from build123d import *

# Parameters (mm, degrees)
F0_W     = 463
F0_H     = 316
F1_DEPTH = 12
F3_DEPTH = 12.001
F4_W     = 408
F4_H     = 10
F4_W_2   = 391
F5_DEPTH = 5.75
F6_R     = 10
F7_R     = 5


with BuildPart() as f1:
    # F0 (on Top) → F1 (new body)
    with BuildSketch(Plane.XY):
        with Locations((231.5, 158)):
            Rectangle(F0_W, F0_H)
    extrude(amount=F1_DEPTH)

    # F2 (on face) → F3 (cut, through all)
    with BuildSketch(Plane.XY.offset(12)):
        with BuildLine():
            Line((395.9189609317, 233.4), (309, 233.4))
            ThreePointArc((309, 233.4), (305.4644660941, 231.9355339059), (304, 228.4))
            Line((304, 228.4), (304, 158))
            ThreePointArc((304, 158), (302.5355339059, 154.4644660941), (299, 153))
            Line((299, 153), (59.3, 153))
            ThreePointArc((59.3, 153), (55.7644660941, 151.5355339059), (54.3, 148))
            Line((54.3, 148), (54.3, 63.8530360718))
            ThreePointArc((54.3, 63.8530360718), (55.7121305741, 60.3706241228), (59.150877193, 58.8552603277))
            Line((59.150877193, 58.8552603277), (111.2746434829, 57.3))
            Line((111.2746434829, 57.3), (299, 57.3))
            ThreePointArc((299, 57.3), (302.5355339059, 55.8355339059), (304, 52.3))
            Line((304, 52.3), (304, 25.3))
            ThreePointArc((304, 25.3), (305.4644660941, 21.7644660941), (309, 20.3))
            Line((309, 20.3), (446, 20.3))
            Line((446, 20.3), (446, 0))
            Line((446, 0), (463, 0))
            Line((463, 0), (463, 20.3))
            Line((463, 20.3), (463, 233.4))
            Line((463, 233.4), (463, 251))
            Line((463, 251), (429.1265081015, 239.0747180711))
            ThreePointArc((429.1265081015, 239.0747180711), (412.7634230352, 234.8288881241), (395.9189609317, 233.4))
        make_face()
    extrude(amount=-F3_DEPTH, mode=Mode.SUBTRACT)

    # F4 (on face) → F5 (cut)
    with BuildSketch(Plane.XY.offset(12)):
        with Locations((259, 311)):
            Rectangle(F4_W, F4_H)
        with Locations((250.5, 5)):
            Rectangle(F4_W_2, F4_H)
    extrude(amount=-F5_DEPTH, mode=Mode.SUBTRACT)

    # F6
    f6_edges = [f1.edges().sort_by_distance(p)[0] for p in [
        (0, 316, 6),
        (0, 0, 6),
        (463, 251, 6),
    ]]
    fillet(f6_edges, radius=F6_R)

    # F7
    f7_edges = [f1.edges().sort_by_distance(p)[0] for p in [
        (446, 20.3, 6),
    ]]
    fillet(f7_edges, radius=F7_R)


solid = f1.part
Input: part model. Units: mm. Frame: model coordinates. A direction names the side the tool comes from. Give positions to 0.01 mm unless a question says otherwise; leave off trailing zeros. Write each loop counter-clockwise with the first axis right and the second up, starting at its lowest first coordinate (ties: lowest second). Pieces come first, ordered by that corner, then holes.
Q1. Section C-C, the plane x = 358.5. Output: boundary loops of the cut face in (y, z).
Q2. Section D-D, the plane y = 111.5. Output: boundary loops of the cut face in (x, z), plus the area to 3 significant figures.
Q3. Set-up query: faces 5 (the face through (256, 311, 6.25)), 6 (the face through (248, 5, 6.25)), 7 (the face through (304, 39, 6)). Return all of +Z, -Z, +X, -X, +Y, -Y with unobstructed straight access to the full face (end or side cutting, diameter ignored); none if empty.
Q4. Pull-direction query (Y, two-part tool) for faces 1 (the face through (413, 234.87, 6.08)), 2 (the face through (204, 57.3, 6)), 3 (the face through (177, 160, 0)), 4 (the face through (461.21, 252.37, 5.92)); classes: pulls with the +Y half, pulls with the -Y half, needs draft (parallel to the pull), parting line crosses it, or undercut.
Q5. Material intervals for probe 1 along Y at (x, z) = (300, 9.5); probe 2 along Y at (x, z) = (252, 10.25); probe 3 along X at (y, z) = (89, 10.5), sorted ascending.
Q6. First-contact query: P1, Ø4.5, axis at y = 5.5, z = 9, coming from the +X side; P2, Ø3, axis at x = 317, y = 311.5, coming from the +Z side; P3, Ø1.5, axis at x = 297, z = 9, coming from the -Y side; P4, Ø6, axis at x = 375.5, z = 8.5, coming from the +Y side. Flat tips, straight axial feed; report the tip coordinate or a pass-through.
Q7. Section A-A, the plane x = 127. Output: boundary loops of the cut face in (y, z).
Filled in:
1. outline: (0, 0) - (20.3, 0) - (20.3, 12) - (10, 12) - (10, 6.25) - (0, 6.25) - close; (233.4, 0) - (316, 0) - (316, 6.25) - (306, 6.25) - (306, 12) - (233.4, 12) - close
2. outline: (0, 0) - (54.3, 0) - (54.3, 12) - (0, 12) - close
2. area: 652 mm2
3. face 5: +Z, +X, +Y
3. face 6: +Z, +X, -Y
3. face 7: +Z, -Z, +X
4. face 1: undercut
4. face 2: undercut
4. face 3: needs draft
4. face 4: pulls with the -Y half
5. probe 1: y = 10 to 57.2, 153.1 to 306
5. probe 2: y = 10 to 57.3, 153 to 306
5. probe 3: x = 0 to 54.3
6. P1: stops at x = 55
6. P2: stops at z = 6.25
6. P3: stops at y = 10
6. P4: stops at y = 316
7. outline: (0, 0) - (57.3, 0) - (57.3, 12) - (10, 12) - (10, 6.25) - (0, 6.25) - close; (153, 0) - (316, 0) - (316, 6.25) - (306, 6.25) - (306, 12) - (153, 12) - close
